Part model, mm, in its own coordinate system. A direction names the side the tool comes from. Coordinates: 2 decimals unless noted, no trailing zeros. Loops run counter-clockwise (first coordinate to the right, second up) from the corner with the lowest first, then second, coordinate; pieces in that order, holes last. Notation, with made-up numbers: M 78,15.5 L 119,15.5 A15 cw 119,44.5 Z; hole C -17.5,22.5 d6. An arc over 180 degrees is marked long. Use a Markdown table: item, result. Add a question column.
1) Band-saw the part on C-C (z = 5.5). List the corners of the cut face in (x, y).
2) Band-saw the part on D-D (x = -26). List the corners of the cut face in (y, z), plus the area to 3 significant figures.
3) Pull direction X, two halves, no side cores. Call faces 4 (the flat face through (-101, 22.633, 9)), 5 (the cylindrical face through (-39.493, 27.854, 13.539)), 6 (the flat face through (20.431, 19, 9)): released by +X, released by -X, zero draft, split by the parting line, or undercut.
4) Pin check, flat tips, straight feed: pin 1 Ø10 at (x, y) = (-24.5, 30) entering from -Z; pin 2 Ø4 at (y, z) = (45, 6.5) entering from -X; pin 3 Ø7.5 at (x, z) = (-73, 8) entering from +Y; pin 4 Ø21 at (x, y) = (-44.57, 37.61) entering from -Z. Stop position of each tip, or through.
5) Tool access for faces 1 (the flat face through (-71, 22.633, 9)), 2 (the flat face through (-109.569, 19, 9)), 3 (the flat face through (12, 22.633, 9)): list every direction of +Z, -Z, +X, -X, +Y, -Y with a clear straight run to the whole face (end or side of a thin tool).
6) Band-saw the part on B-B (x = -69). List the corners of the cut face in (y, z), plus the area to 3 significant figures.
7) Band-saw the part on A-A (z = 12.5). List the corners of the cut face in (x, y).
8) Wall check: probe 1 along X at (y, z) = (24.5, 14); probe 2 along X at (y, z) = (27.5, 12); probe 3 along Y at (x, z) = (-68, 5.75). Give the ranges that are in metal, low to high. Write a range as from..to.
from build123d import *

# Parameters (mm, degrees)
F0_W     = 32
F0_H     = 7
F0_H_2   = 29
F0_R     = 13
F0_R_2   = 11
F1_DEPTH = 18
F2_D     = 26
F2_DEPTH = 8
F2_TIP   = 7.8111880474
F3_R     = 6


with BuildPart() as f1:
    # F0 (on Top) → F1 (new body)
    with BuildSketch(Plane.XY):
        with Locations((-44.5692668381, 19.1334804479)):
            Rectangle(F0_W, F0_H)
        with Locations((-44.5692668381, 37.1334804479)):
            Rectangle(F0_W, F0_H_2)
        with Locations((-44.5691263461, 37.6129510462)):
            Circle(F0_R, mode=Mode.SUBTRACT)
        Polygon((-92.0692668381, 22.6334804479), (-109.5692668381, 22.6334804479), (-109.5692668381, 15.6334804479), (-60.5692668381, 15.6334804479), (-60.5692668381, 22.6334804479), (-76.0692668381, 22.6334804479), (-81.0692668381, 22.6334804479), (-87.0692668381, 22.6334804479), align=None)
        Polygon((-13.0689858541, 22.6334804479), (-28.5692668381, 22.6334804479), (-28.5692668381, 15.6334804479), (20.4307331619, 15.6334804479), (20.4307331619, 22.6334804479), (3.0333849776, 22.6334804479), (-1.9666150224, 22.6334804479), (-8.0689858541, 22.6334804479), align=None)
        with Locations((-44.5691263461, 37.6129510462)):
            Circle(F0_R)
        with Locations((-44.5691263461, 37.6129510462)):
            Circle(F0_R_2, mode=Mode.SUBTRACT)
        Polygon((-81.0692668381, 22.6334804479), (-76.0692668381, 22.6334804479), (-81.0692668381, 30.2172819608), align=None)
        with BuildLine():
            Line((-87.0692668381, 30.2172819608), (-87.0692668381, 22.6334804479))
            Line((-87.0692668381, 22.6334804479), (-81.0692668381, 22.6334804479))
            Line((-81.0692668381, 22.6334804479), (-81.0692668381, 30.2172819608))
            ThreePointArc((-81.0692668381, 30.2172819608), (-84.0692668381, 29.6334804479), (-87.0692668381, 30.2172819608))
        make_face()
        Polygon((-87.0692668381, 30.2172819608), (-92.0692668381, 22.6334804479), (-87.0692668381, 22.6334804479), align=None)
        Polygon((-8.0689858541, 30.2171683033), (-13.0689858541, 22.6334804479), (-8.0689858541, 22.6334804479), align=None)
        with BuildLine():
            Line((-8.0689858541, 30.2171683033), (-8.0689858541, 22.6334804479))
            Line((-8.0689858541, 22.6334804479), (-1.9666150224, 22.6334804479))
            Line((-1.9666150224, 22.6334804479), (-2.018655908, 30.2379566021))
            ThreePointArc((-2.018655908, 30.2379566021), (-5.0417798399, 29.633527669), (-8.0689858541, 30.2171683033))
        make_face()
        Polygon((-1.9666150224, 22.6334804479), (3.0333849776, 22.6334804479), (-2.018655908, 30.2379566021), align=None)
    extrude(amount=F1_DEPTH)

    # F2
    with Locations(Plane(origin=(0, 0, 0), x_dir=(1, 0, 0), z_dir=(0, 0, -1))):
        with Locations((-44.5691263461, -37.6129510462)):
            Hole(F2_D / 2, depth=F2_DEPTH)
            with Locations((0, 0, -(F2_DEPTH + F2_TIP / 2))):  # 118° drill point
                Cone(0, F2_D / 2, F2_TIP, mode=Mode.SUBTRACT)

    # F3
    f3_edges = [f1.edges().sort_by_distance(p)[0] for p in [
        (-60.569267, 22.63348, 9),
        (-28.569267, 22.63348, 9),
        (-60.569267, 51.63348, 9),
        (-28.569267, 51.63348, 9),
    ]]
    fillet(f3_edges, radius=F3_R)


solid = f1.part
Entries:
| question | item | result |
|---|---|---|
| 1 | outline | M -109.57,15.63 L 20.43,15.63 L 20.43,22.63 L 3.03,22.63 L -2.02,30.24 A8 cw -8.07,30.22 L -13.07,22.63 L -22.57,22.63 A6 cw -28.57,28.63 L -28.57,45.63 A6 ccw -34.57,51.63 L -54.57,51.63 A6 ccw -60.57,45.63 L -60.57,28.63 A6 cw -66.57,22.63 L -76.07,22.63 L -81.07,30.22 A8 cw -87.07,30.22 L -92.07,22.63 L -109.57,22.63 Z; hole C -44.57,37.61 d26 |
| 2 | outline | M 15.63,0 L 23.71,0 L 23.71,18 L 15.63,18 Z |
| 2 | area | 145 mm2 |
| 3 | face 4 | zero draft |
| 3 | face 5 | undercut |
| 3 | face 6 | released by +X |
| 4 | pin 1 | z = 0 |
| 4 | pin 2 | x = -60.57 |
| 4 | pin 3 | y = 23.67 |
| 4 | pin 4 | through |
| 5 | face 1 | +Z, -Z, +Y |
| 5 | face 2 | +Z, -Z, -X, +Y, -Y |
| 5 | face 3 | +Z, -Z, +X, +Y |
| 6 | outline | M 15.63,0 L 22.63,0 L 22.63,18 L 15.63,18 Z |
| 6 | area | 126 mm2 |
| 7 | outline | M -109.57,15.63 L 20.43,15.63 L 20.43,22.63 L 3.03,22.63 L -2.02,30.24 A8 cw -8.07,30.22 L -13.07,22.63 L -22.57,22.63 A6 cw -28.57,28.63 L -28.57,45.63 A6 ccw -34.57,51.63 L -54.57,51.63 A6 ccw -60.57,45.63 L -60.57,28.63 A6 cw -66.57,22.63 L -76.07,22.63 L -81.07,30.22 A8 cw -87.07,30.22 L -92.07,22.63 L -109.57,22.63 Z; hole C -44.57,37.61 d22 |
| 8 | probe 1 | -90.84..-77.3, -62.22..-26.92, -11.84..1.79 |
| 8 | probe 2 | -88.86..-79.28, -60.68..-48.9, -40.24..-28.46, -9.86..-0.2 |
| 8 | probe 3 | 15.63..22.63 |
